Check sheet for the modelled part. Datum: model origin and axes. Units: mm. A direction names the side the tool comes from. Give positions to 0.01 mm unless a question says otherwise; leave off trailing zeros. Write each loop counter-clockwise with the first axis right and the second up, starting at its lowest first coordinate (ties: lowest second). Pieces come first, ordered by that corner, then holes. Notation, with made-up numbers: M 65.5,9 L 105.5,9 A7 cw 105.5,16 Z; hole C -10,38.25 d1. An arc over 180 degrees is marked long. Write item = value, one per line. Start each with the question number.
1) Mould release check, pull along X, two halves, no side actions. Record for faces 4 (the flat face through (36.8, 20.7, 5.9)), 5 (the cylindrical face through (32.5, 5.5, 3)), 6 (the flat face through (33, 10, 9)): released by +X, released by -X, zero draft, split by the parting line, or undercut.
2) Scan lines: line 1 along X through (y, z) = (17.5, 6); line 2 along Y through (x, z) = (32.5, 6.75); line 3 along Z through (x, y) = (28.5, 5). Record each from-to range of solid material in increasing order. Write a range as [from, to].
3) Cross-section at D-D, the plane x = 32.5. Record the cut outline in (y, z).
4) Cross-section at A-A, the plane x = 4. Record the cut outline in (y, z), plus the area to 3 significant figures.
5) Access from +Z, -Z, +X, -X, +Y, -Y to the whole of each face (thin tool, end or side, straight path). Record for faces 1 (the flat face through (32, 6, 6)), 2 (the flat face through (13, 14.5, 3)), 3 (the flat face through (34.5, 2, 3)).
6) Go/stop test with flat-tipped pins: pin 1 (1.8 mm diameter, centred on x = 32, z = 8, fed in from -Y); pin 2 (1 mm diameter, centred on y = 1.5, z = 4.5, fed in from -X); pin 3 (3 mm diameter, centred on x = 33.5, y = 3.5, fed in from +Z); pin 4 (1.9 mm diameter, centred on x = 4, z = 6, fed in from +Y). Record where each tip stops, or that it passes through.
7) Cross-section at B-B, the plane y = 18. Record the cut outline in (x, z), plus the area to 3 significant figures.
8) Cross-section at C-C, the plane z = 1.25. Record the cut outline in (x, y), plus the area to 3 significant figures.
Autodesk Inventor part; units mm, degrees
ref_plane "body_XY" through (32.5, 18, 6) normal (0, 0, 1) x (1, 0, 0)
ref_plane "body_YZ" through (32.5, 18, 6) normal (1, 0, 0) x (0, 1, 0)
ref_plane "body_ZX" through (32.5, 18, 6) normal (0, 1, 0) x (0, 0, 1)
sketch "Sketch_1" plane through (0, 0, 0) normal (0, 0, 1) x (1, 0, 0)
  line L0 (0, 14.5) -> (26, 14.5)
  arc A0 (27.5, 13) -> (26, 14.5) centre (26, 13) ccw
  line L1 (27.5, 13) -> (27.5, 0)
  line L2 (27.5, 0) -> (30.5, 0)
  line L3 (30.5, 0) -> (30.5, 3.5)
  arc A1 (34.5, 3.5) -> (30.5, 3.5) centre (32.5, 3.5) ccw
  line L4 (34.5, 3.5) -> (34.5, 0)
  line L5 (34.5, 0) -> (37.5, 0)
  line L6 (37.5, 0) -> (37.5, 20)
  line L7 (37.5, 20) -> (36, 21.5)
  line L8 (36, 21.5) -> (0, 21.5)
  line L9 (0, 21.5) -> (0, 14.5)
extrude "Extrusion1" add sketch "Sketch_1" along normal blind 12
sketch "Sketch2" plane through (0, 0, 0) normal (0, 0, -1) x (-1, 0, 0)
  point P0 (-32.5, 18)
hole "Hole1" at (32.5, 18, 0) direction (0, 0, 1) diameter 4 depth 12
sketch "Sketch_3" plane through (4, 0, 0) normal (1, 0, 0) x (0, 0, -1)
  line L0 (-6, 14.5) -> (-6, 21.5)
  line L1 (-6, 21.5) -> (-4, 21.5)
  line L2 (-4, 21.5) -> (-4.379, 21.121)
  line L3 (-4.379, 21.121) -> (-4.379, 14.879)
  line L4 (-4.379, 14.879) -> (-4, 14.5)
  line L5 (-4, 14.5) -> (-6, 14.5)
  line L6 (-6, 14.5) -> (-6, 21.5)
revolve "Revolution1" cut sketch "Sketch_3" angle 360 about axis through (4, 14.5, 6) along (0, -1, 0)
thread "Thread1"
sketch "Sketch_4" plane through (14, 0, 0) normal (1, 0, 0) x (0, 0, -1)
  line L0 (-6, 14.5) -> (-6, 21.5)
  line L1 (-6, 21.5) -> (-4, 21.5)
  line L2 (-4, 21.5) -> (-4.379, 21.121)
  line L3 (-4.379, 21.121) -> (-4.379, 14.879)
  line L4 (-4.379, 14.879) -> (-4, 14.5)
  line L5 (-4, 14.5) -> (-6, 14.5)
  line L6 (-6, 14.5) -> (-6, 21.5)
revolve "Revolution2" cut sketch "Sketch_4" angle 360 about axis through (14, 14.5, 6) along (0, -1, 0)
thread "Thread2"
sketch "Sketch_6" plane through (0, 0, 6) normal (0, 0, 1) x (1, 0, 0)
  line L0 (27.5, 0) -> (37.5, 0)
  line L1 (37.5, 0) -> (37.5, 10)
  line L2 (37.5, 10) -> (27.5, 10)
  line L3 (27.5, 10) -> (27.5, 0)
extrude "Extrusion2" cut sketch "Sketch_6" along normal blind 6
ref_plane "body_XY" through (32.5, 18, 6) normal (0, 0, 1) x (1, 0, 0)
ref_plane "body_YZ" through (32.5, 18, 6) normal (1, 0, 0) x (0, 1, 0)
ref_plane "body_ZX" through (32.5, 18, 6) normal (0, 1, 0) x (0, 0, 1)
properties part number "MCHA-20_(g)"
Reply:
q1.face_4 = released by +X
q1.face_5 = undercut
q1.face_6 = zero draft
q2.line_1 = [0, 2.38], [5.62, 12.38], [15.62, 30.56], [34.44, 37.5]
q2.line_2 = [10, 16], [20, 21.5]
q2.line_3 = [0, 6]
q3.outline = M 5.5,0 L 16,0 L 16,12 L 10,12 L 10,6 L 5.5,6 Z; M 20,0 L 21.5,0 L 21.5,12 L 20,12 Z
q4.outline = M 14.5,0 L 21.5,0 L 21.5,4 L 21.12,4.38 L 14.88,4.38 L 14.5,4 Z; M 14.5,8 L 14.88,7.62 L 21.12,7.62 L 21.5,8 L 21.5,12 L 14.5,12 Z
q4.area = 61.0 mm2
q5.face_1 = +Z, +X, -X, -Y
q5.face_2 = +Z, -Z, -X, -Y
q5.face_3 = +Z, -Z, -Y
q6.pin_1 = 10
q6.pin_2 = 27.5
q6.pin_3 = 6
q6.pin_4 = through
q7.outline = M 0,0 L 30.5,0 L 30.5,12 L 0,12 Z; M 34.5,0 L 37.5,0 L 37.5,12 L 34.5,12 Z; hole C 4,6 d3.24; hole C 14,6 d3.24
q7.area = 385 mm2
q8.outline = M 0,14.5 L 26,14.5 A1.5 cw 27.5,13 L 27.5,0 L 30.5,0 L 30.5,3.5 A2 cw 34.5,3.5 L 34.5,0 L 37.5,0 L 37.5,20 L 36,21.5 L 0,21.5 Z; hole C 32.5,18 d4
q8.area = 374 mm2
